Geometry check sheet. Reference: the model listing, model coordinates, mm. Face numbers are marked on the shaded views. Give positions to 0.01 mm unless a question says otherwise; leave off trailing zeros. Put each result on its own line as item: value. Start each with the question number.
Q1. Section check A-A on y = 0. State how many separate pieces and enclosed holes the cut face has, then the cut area to 3 significant figures.
Q2. Mould release check, pull along X, two halves, no side actions. Record for the marked faces 1 and 2: +X half, -X half, draft (parallel to the pull), parting line (faces both ways), or undercut.
Q3. Material ranges on L1, parallel to Y at x = 60, z = 20.25; L2, parallel to X at y = 27, z = 9.75; L3, parallel to Y at x = 60, z = 22, recorded low to high.
Q4. Go/stop test with flat-tipped pins: pin 1 (1.5 mm diameter, centred on y = 36.5, z = 20.5, fed in from +X); pin 2 (6 mm diameter, centred on y = 6.5, z = 21, fed in from +X); pin 3 (2 mm diameter, centred on x = 3, z = 24, fed in from -Y). Record where each tip stops, or that it passes through.
```python
from build123d import *

# Parameters (mm, degrees)
SKETCH1_R           = 125
BOSS_EXTRUDE1_DEPTH = 30
FILLET1_R           = 15
SKETCH2_R           = 15
CUT_EXTRUDE1_DEPTH  = 30
SKETCH3_R           = 30
SKETCH3_R_2         = 15
CUT_EXTRUDE2_DEPTH  = 50


with BuildPart() as part:
    # Sketch1 → Boss-Extrude1 (new body)
    with BuildSketch(Plane.XY):
        Circle(SKETCH1_R)
    extrude(amount=BOSS_EXTRUDE1_DEPTH)

    # Fillet1
    fillet1_edges = [part.edges().sort_by_distance(p)[0] for p in [
        (-125, 0, 0),
        (-125, 0, 30),
    ]]
    fillet(fillet1_edges, radius=FILLET1_R - 0.0001)  # a hair under: the kernel refuses the full size

    # Sketch2 → Cut-Extrude1 (cut)
    with BuildSketch(Plane.XY.offset(30)):
        Circle(SKETCH2_R)
    extrude(amount=-CUT_EXTRUDE1_DEPTH, mode=Mode.SUBTRACT)

    # Sketch3 → Cut-Extrude2 (cut)
    with BuildSketch(Plane.XY.offset(30)):
        with Locations((0, 60)):
            Circle(SKETCH3_R)
        with Locations((-60, 0)):
            Circle(SKETCH3_R)
        with Locations((0, -60)):
            Circle(SKETCH3_R)
        with Locations((60, 0)):
            Circle(SKETCH3_R)
        with Locations((55, -55)):
            Circle(SKETCH3_R_2)
        with Locations((-55, -55)):
            Circle(SKETCH3_R_2)
        with Locations((-55, 55)):
            Circle(SKETCH3_R_2)
        with Locations((55, 55)):
            Circle(SKETCH3_R_2)
    extrude(amount=-CUT_EXTRUDE2_DEPTH, mode=Mode.SUBTRACT)


solid = part.part
```
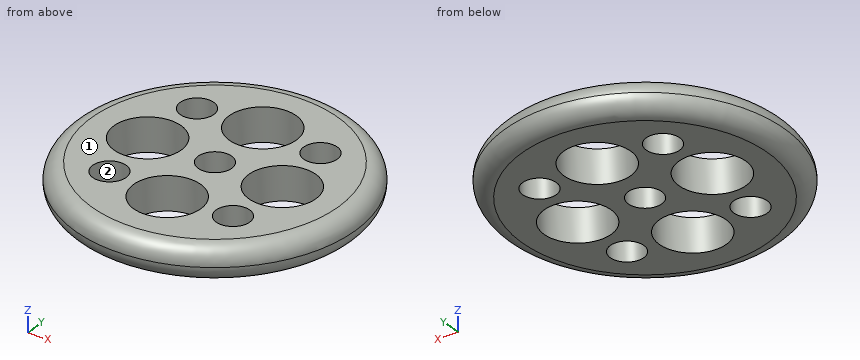
Results found:
1. separate pieces: 4
1. enclosed holes: 0
1. area: 2,810 mm^2
2. face 1: draft
2. face 2: undercut
3. L1: y = -108.58 to -69.14, -40.86 to -30, 30 to 40.86, 69.14 to 108.58
3. L2: x = -121.08 to -73.08, -46.92 to 46.92, 73.08 to 121.08
3. L3: y = -107.68 to -69.14, -40.86 to -30, 30 to 40.86, 69.14 to 107.68
4. pin 1: stops at x = 118.83
4. pin 2: stops at x = 124.54
4. pin 3: stops at y = -122.65
